```python
from build123d import *

# Parameters (mm, degrees)
TUBE_SQUARE_RHS50X50X5_1_DEPTH = 700


with BuildPart() as part:
    # Sketch1 → Tube (square) RHS50X50X5(1) (new body)
    with BuildSketch(Plane.YZ):
        with BuildLine():
            Line((-15, -25), (15, -25))
            ThreePointArc((15, -25), (22.071067812, -22.071067812), (25, -15))
            Line((25, -15), (25, 15))
            ThreePointArc((25, 15), (22.071067812, 22.071067812), (15, 25))
            Line((15, 25), (-15, 25))
            ThreePointArc((-15, 25), (-22.071067812, 22.071067812), (-25, 15))
            Line((-25, 15), (-25, -15))
            ThreePointArc((-25, -15), (-22.071067812, -22.071067812), (-15, -25))
        make_face()
        with BuildLine():
            Line((-15, -20), (15, -20))
            ThreePointArc((15, -20), (18.535533906, -18.535533906), (20, -15))
            Line((20, -15), (20, 15))
            ThreePointArc((20, 15), (18.535533906, 18.535533906), (15, 20))
            Line((15, 20), (-15, 20))
            ThreePointArc((-15, 20), (-18.535533906, 18.535533906), (-20, 15))
            Line((-20, 15), (-20, -15))
            ThreePointArc((-20, -15), (-18.535533906, -18.535533906), (-15, -20))
        make_face(mode=Mode.SUBTRACT)
    extrude(amount=TUBE_SQUARE_RHS50X50X5_1_DEPTH)


solid = part.part
```
The listing builds one solid part. Answer for the finished solid, in the listing's coordinates (mm). A direction names the side the tool comes from. Give positions to 0.01 mm unless a question says otherwise; leave off trailing zeros. Order: outer loops, then holes, each group sorted by start corner. A loop starts at its lowest first (then second) coordinate and runs counter-clockwise, first axis right, second up. Notation, with made-up numbers: (-0.5, 81) -> (46.5, 81) arc R17 ccw to (46.5, 97) -> close; hole circle Ø6 at (72.5, 35.25). An arc over 180 degrees is marked (long way). Answer as a JSON object with one key per item and string values. Group by question number.
Item 1: The part is cut by section C-C on x = 267.5. Write down the section's boundary in (y, z), and give its area (3 significant figures).
Item 2: Consider L1, parallel to Y at x = 624.5, z = 12; L2, parallel to Z at x = 481.5, y = -17. Determine where each line is inside the solid, lowest interval first. Write a range as from..to.
Item 3: A flat-ended cylindrical pin translates along its axis: pin 1 (4 mm diameter, centred on x = 299.5, z = -17.5, fed in from -Y). Find the tip coordinate at first contact, or state that the pin passes through.
Item 4: A tool of negligible diameter and unlimited length cuts with its end or side. For faces 1 (the flat face through (345, -25, 0)), 2 (the flat face through (345, 0, -20)), from which of +Z, -Z, +X, -X, +Y, -Y can it reach the whole face along a straight path? Write none if from no direction.
Item 5: The part is cut by section A-A on z = 6. Write down the section's boundary in (x, y), and give its area (3 significant figures).
Item 6: Determine the mould class of faces 3 (the flat face through (345, 20, 0)), 4 (the flat face through (345, 25, 0)), 5 (the flat face through (345, 0, -25)) for opening direction Z: pulls with the +Z half, pulls with the -Z half, needs draft (parallel to the pull), parting line crosses it, or undercut.
Result set:
{
 "1": {"outline": "(-25, -15) arc R10 ccw to (-15, -25) -> (15, -25) arc R10 ccw to (25, -15) -> (25, 15) arc R10 ccw to (15, 25) -> (-15, 25) arc R10 ccw to (-25, 15) -> close; hole (-20, -15) arc R5 ccw to (-15, -20) -> (15, -20) arc R5 ccw to (20, -15) -> (20, 15) arc R5 ccw to (15, 20) -> (-15, 20) arc R5 ccw to (-20, 15) -> close", "area": "836 mm²"},
 "2": {"L1": "-25..-20, 20..25", "L2": "-24.8..-19.58, 19.58..24.8"},
 "3": {"pin 1": "y = -24.99"},
 "4": {"face 1": "+Z, -Z, +X, -X, -Y", "face 2": "+X, -X"},
 "5": {"outline": "(0, -25) -> (700, -25) -> (700, -20) -> (0, -20) -> close; (0, 20) -> (700, 20) -> (700, 25) -> (0, 25) -> close", "area": "7,000 mm²"},
 "6": {"face 3": "undercut", "face 4": "needs draft", "face 5": "pulls with the -Z half"}
}
